```python
from build123d import *

# Parameters (mm, degrees)
F0_W   = 14.5
F0_H   = 5.4750965592
F0_W_2 = 5
F3_D   = 3
F4_R   = 1.5


with BuildPart() as f1:
    # F0 (on Front) → F1 (revolve)
    with BuildSketch(Plane.XZ):
        with Locations((24.75, 2.7375482796)):
            Rectangle(F0_W, F0_H)
        Polygon((12.5, 35), (12.5, 5.4750965592), (17.5, 5.4750965592), (17.5, 35), (16, 35), (16, 33.9), (14, 33.9), (14, 35), align=None)
        with Locations((15, 2.7375482796)):
            Rectangle(F0_W_2, F0_H)
    revolve(axis=Axis((0, 0, 26.583340019), (0, 0, 1)))

    # F3 (through all)
    with Locations(Plane(origin=(0, 0, 0), x_dir=(1, 0, 0), z_dir=(0, 0, -1))):
        with Locations((0, -28.5), (28.5, 0), (0, 28.5), (-28.5, 0)):
            Hole(F3_D / 2)

    # F4
    f4_edges = [f1.edges().sort_by_distance(p)[0] for p in [
        (-32, 0, 5.475097),
    ]]
    fillet(f4_edges, radius=F4_R)


solid = f1.part
```
Part model, mm, in its own coordinate system. A direction names the side the tool comes from. Coordinates: 2 decimals unless noted, no trailing zeros. Write each loop counter-clockwise with the first axis right and the second up, starting at its lowest first coordinate (ties: lowest second). Pieces come first, ordered by that corner, then holes.
Item 1: Which spindle directions (+Z, -Z, +X, -X, +Y, -Y) get a long thin tool onto all of the face, cutting with end or side? Do faces 4 (the face through (-27, 0, 3)), 5 (the face through (-3.47, -15.62, 34.44)). Say none if no direction does.
Item 2: Mould opens along Y. For faces 1 (the face through (-13.887, -10.648, 20.444)), 2 (the face through (-0.07, -14.15, 33.9)), 3 (the face through (-13, -13, 5.475)) say: released by +Y, released by -Y, zero draft, split by the parting line, or undercut.
Item 3: Slice it at A-A (y = 0). Count the separate pieces of the cut face and the enclosed holes in it, and give its area (3 significant figures).
Item 4: Pin check, flat tips, straight feed: pin 1 (4 mm diameter, centred on x = 9.5, y = -18.5, fed in from -Z); pin 2 (2 mm diameter, centred on x = -24, z = 5.5, fed in from -Y); pin 3 (5 mm diameter, centred on y = 5, z = 10.5, fed in from +X); pin 4 (10 mm diameter, centred on x = 19, y = -18, fed in from +Z). Stop position of each tip, or through.
Item 5: Slice it at C-C (z = 26). Write the cut outline in (x, y), and give its area (3 significant figures).
Item 6: Probe line 1 (Z direction, x = 24, y = -16); line 2 (X direction, y = -1.5, z = 29.5); line 3 (X direction, y = -0.5, z = 19). List the from-to ranges inside material, lowest first.
Results found:
1. face 4: +Z, -Z
1. face 5: +Z
2. face 1: split by the parting line
2. face 2: undercut
2. face 3: zero draft
3. separate pieces: 4
3. enclosed holes: 0
3. area: 471 mm2
4. pin 1: stops at z = 0
4. pin 2: stops at y = -21.59
4. pin 3: stops at x = 17.32
4. pin 4: stops at z = 5.48
5. outline: circle Ø35 at (0, 0); hole circle Ø25 at (0, 0)
5. area: 471 mm2
6. line 1: z = 0 to 5.48
6. line 2: x = -17.44 to -12.41, 12.41 to 17.44
6. line 3: x = -17.49 to -12.49, 12.49 to 17.49
